```python
from build123d import *

# Parameters (mm, degrees)
F1_DEPTH  = 16
F2_W      = 17.5
F2_H      = 20
F3_DEPTH  = 13
F5_DEPTH  = 0.6
F7_DEPTH  = 1.6
F9_D      = 2.6
F10_W     = 15
F10_H     = 4.3693144321
F11_DEPTH = 7


with BuildPart() as f1:
    # F0 (on Top) → F1 (new body)
    with BuildSketch(Plane.XY):
        Polygon((15, 23), (0, 23), (0, 0), (22.5, 0), (22.5, 28), (0, 28), (0, 26), (15, 26), align=None)
    extrude(amount=F1_DEPTH)

    # F2 (on face) → F3 (cut)
    with BuildSketch(Plane.XY.offset(16)):
        with Locations((8.75, 10)):
            Rectangle(F2_W, F2_H)
    extrude(amount=-F3_DEPTH, mode=Mode.SUBTRACT)

    # F4 (on face) → F5 (cut)
    with BuildSketch(Plane.XY.offset(16)):
        with BuildLine():
            Line((17.5, 22.25), (0, 22.25))
            Line((0, 22.25), (0, 21.25))
            Line((0, 21.25), (17.5, 21.25))
            ThreePointArc((17.5, 21.25), (18.3838834765, 20.8838834765), (18.75, 20))
            Line((18.75, 20), (18.75, 0))
            Line((18.75, 0), (19.75, 0))
            Line((19.75, 0), (19.75, 20))
            ThreePointArc((19.75, 20), (19.0909902577, 21.5909902577), (17.5, 22.25))
        make_face()
    extrude(amount=-F5_DEPTH, mode=Mode.SUBTRACT)

    # F6 (on face) → F7 (cut)
    with BuildSketch(Plane(origin=(0, 0, 0), x_dir=(1, 0, 0), z_dir=(0, 0, -1))):
        Polygon((19.9547005384, -26.5), (21.1094010768, -24.5), (19.9547005384, -22.5), (17.6452994616, -22.5), (16.4905989232, -24.5), (17.6452994616, -26.5), align=None)
    extrude(amount=-F7_DEPTH, mode=Mode.SUBTRACT)

    # F9 (through all)
    with Locations(Plane(origin=(0, 0, 0), x_dir=(1, 0, 0), z_dir=(0, 0, -1))):
        with Locations((18.8, -24.5)):
            Hole(F9_D / 2)

    # F10 (on face) → F11 (cut)
    with BuildSketch(Plane.XY.offset(16)):
        with Locations((7.5, 28.1846572161)):
            Rectangle(F10_W, F10_H)
    extrude(amount=-F11_DEPTH, mode=Mode.SUBTRACT)

    # F12: F1 across plane


with BuildPart() as f1_1:
    add(f1.part)
    add(f1.part.mirror(Plane.YZ))

    # F13: F1 across plane


with BuildPart() as f1_2:
    add(f1_1.part)
    add(f1_1.part.mirror(Plane.XZ))


solid = f1_2.part
```
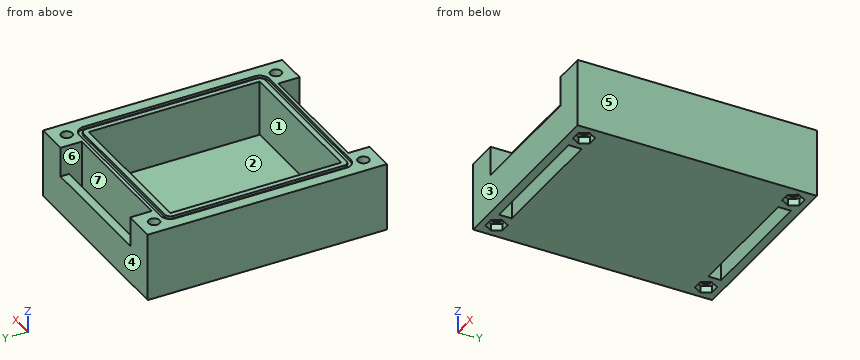
Work out the finished part from the listing and answer in its coordinate system (mm). Face numbers are marked on the shaded views. A direction names the side the tool comes from. Coordinates: 2 decimals unless noted, no trailing zeros. Order: outer loops, then holes, each group sorted by start corner. A loop starts at its lowest first (then second) coordinate and runs counter-clockwise, first axis right, second up. Notation, with made-up numbers: M 83.25,56 L 124.25,56 A15 cw 124.25,76 Z; hole C -22,-33.5 d6. An arc over 180 degrees is marked long. Use CSV: the item, a comma, the result in double quotes.
1) Consider line 1 (X direction, y = 24.5, z = 5.75); line 2 (Y direction, x = -7, z = 5.5); line 3 (Y direction, x = 18.8, z = 5.25). Determine where each line is inside the solid, lowest interval first. Write a range as [from, to].
Worked out:
line 1,"x = [-22.5, -20.1], [-17.5, -15], [15, 17.5], [20.1, 22.5]"
line 2,"y = [-28, -26], [-23, -20], [20, 23], [26, 28]"
line 3,"y = [-28, -25.8], [-23.2, 23.2], [25.8, 28]"
2) Flat-ended cylindrical pins translate along their axes: pin 1 Ø1 at (x, y) = (0, -21) entering from -Z; pin 2 Ø1 at (x, y) = (4, 16.5) entering from +Z; pin 3 Ø2 at (x, y) = (18.5, -24) entering from -Z. Find the tip coordinate at first contact, or state that the pin passes through.
Worked out:
pin 1,"stops at z = 0"
pin 2,"stops at z = 3"
pin 3,"stops at z = 1.6"
3) For the marked faces 5, 6 and 7, determine the directions among +Z, -Z, +X, -X, +Y, -Y from which every point of the face is accessible in a straight line to the end or side of a thin tool.
Worked out:
face 5,"+Z, -Z, +X, +Y, -Y"
face 6,"+Z"
face 7,"+Z, -Z"
4) Section C-C on y = 8.5 is taken. Write down the section's boundary in (x, z), plus the area to 3 significant figures.
Worked out:
outline,"M -22.5,0 L 22.5,0 L 22.5,16 L 19.75,16 L 19.75,15.4 L 18.75,15.4 L 18.75,16 L 17.5,16 L 17.5,3 L -17.5,3 L -17.5,16 L -18.75,16 L -18.75,15.4 L -19.75,15.4 L -19.75,16 L -22.5,16 Z"
area,"264 mm^2"
5) Section B-B on z = 11.75 is taken. Write down the section's boundary in (x, y).
Worked out:
outline,"M -22.5,-28 L -15,-28 L -15,-23 L 15,-23 L 15,-28 L 22.5,-28 L 22.5,28 L 15,28 L 15,23 L -15,23 L -15,28 L -22.5,28 Z; hole C -18.8,-24.5 d2.6; hole C -18.8,24.5 d2.6; hole M -17.5,-20 L 17.5,-20 L 17.5,20 L -17.5,20 Z; hole C 18.8,-24.5 d2.6; hole C 18.8,24.5 d2.6"
6) Determine the mould class of the marked faces 1, 2, 3 and 4 for opening direction Y: released by +Y, released by -Y, zero draft, split by the parting line, or undercut.
Worked out:
face 1,"undercut"
face 2,"undercut"
face 3,"released by -Y"
face 4,"released by +Y"
7) Section D-D on z = 4.5 is taken. Write down the section's boundary in (x, y), plus the area to 3 significant figures.
Worked out:
outline,"M -22.5,-28 L 22.5,-28 L 22.5,28 L -22.5,28 Z; hole C -18.8,-24.5 d2.6; hole C -18.8,24.5 d2.6; hole M -17.5,-20 L 17.5,-20 L 17.5,20 L -17.5,20 Z; hole M -15,-26 L 15,-26 L 15,-23 L -15,-23 Z; hole M -15,23 L 15,23 L 15,26 L -15,26 Z; hole C 18.8,-24.5 d2.6; hole C 18.8,24.5 d2.6"
area,"919 mm^2"
8) Section A-A on x = -4 is taken. Write down the section's boundary in (y, z).
Worked out:
outline,"M -28,0 L -26,0 L -26,9 L -28,9 Z; M -23,0 L 23,0 L 23,16 L 22.25,16 L 22.25,15.4 L 21.25,15.4 L 21.25,16 L 20,16 L 20,3 L -20,3 L -20,16 L -21.25,16 L -21.25,15.4 L -22.25,15.4 L -22.25,16 L -23,16 Z; M 26,0 L 28,0 L 28,9 L 26,9 Z"
